```python
from build123d import *

# Parameters (mm, degrees)
SKETCH_1_W          = 123
SKETCH_1_H          = 80
EXTRUDE_1_DEPTH     = 93
SHELL_1_T           = -3
SKETCH_2_W          = 50
SKETCH_2_H          = 117
CUT_EXTRUDE_1_DEPTH = 138.227001716
FILLET_1_R          = 5
FILLET_2_R          = 5
CUT_EXTRUDE_2_REACH = 161.305
CUT_EXTRUDE_4_REACH = 161.305
SKETCH_5_W          = 30
SKETCH_5_H          = 56
CUT_EXTRUDE_5_REACH = 120.454
SKETCH_6_R          = 10
FILLET_3_R          = 5
CUT_EXTRUDE_6_REACH = 120.454
SKETCH_7_W          = 5
SKETCH_7_H          = 28


with BuildPart() as part:
    # 草圖1 → 填料-伸長1 (new body)
    with BuildSketch(Plane(origin=(0, 0, 0), x_dir=(0, 0, -1), z_dir=(1, 0, 0))):
        Rectangle(SKETCH_1_W, SKETCH_1_H)
    extrude(amount=EXTRUDE_1_DEPTH)

    # 薄殼1
    shell_1_openings = [part.faces().sort_by_distance(p)[0] for p in [
        (93, 0, 0),
    ]]
    offset(amount=SHELL_1_T, openings=shell_1_openings, kind=Kind.INTERSECTION)

    # 草圖2 → 除料-伸長1 (cut, through all)
    with BuildSketch(Plane(origin=(0, 40, 0), x_dir=(1, 0, 0), z_dir=(0, 1, 0))):
        with Locations((68, 0)):
            Rectangle(SKETCH_2_W, SKETCH_2_H)
    extrude(amount=-CUT_EXTRUDE_1_DEPTH, mode=Mode.SUBTRACT)

    # 圓角1
    fillet_1_edges = [part.edges().sort_by_distance(p)[0] for p in [
        (0, -40, 0),
        (0, 40, 0),
    ]]
    fillet(fillet_1_edges, radius=FILLET_1_R)

    # 圓角2
    fillet_2_edges = [part.edges().sort_by_distance(p)[0] for p in [
        (93, -40, 60),
        (93, -40, -60),
        (93, 40, 60),
        (93, 40, -60),
    ]]
    fillet(fillet_2_edges, radius=FILLET_2_R)

    # 草圖3 → 除料-伸長2 (cut, up to next)
    with BuildSketch(Plane(origin=(0, 0, -61.5), x_dir=(-1, 0, 0), z_dir=(0, 0, -1)), mode=Mode.PRIVATE) as cut_extrude_2_sk1:
        with BuildLine():
            Line((-76.5, -25), (-76.5, 25))
            ThreePointArc((-76.5, 25), (-74, 27.5), (-71.5, 25))
            Line((-71.5, 25), (-71.5, -25))
            ThreePointArc((-71.5, -25), (-74, -27.5), (-76.5, -25))
        make_face()
    cut_extrude_2_tool1 = extrude(cut_extrude_2_sk1.sketch, amount=-CUT_EXTRUDE_2_REACH, mode=Mode.PRIVATE) & part.part
    cut_extrude_2 = cut_extrude_2_tool1.solids().sort_by_distance((74, 0, -61.5))[0]
    add(cut_extrude_2, mode=Mode.SUBTRACT)

    # 鏡射1: 除料-伸長2 across plane
    add(cut_extrude_2.mirror(Plane.XY), mode=Mode.SUBTRACT)

    # 草圖5 → 除料-伸長4 (cut, up to next)
    with BuildSketch(Plane(origin=(0, 0, -61.5), x_dir=(-1, 0, 0), z_dir=(0, 0, -1)), mode=Mode.PRIVATE) as cut_extrude_4_sk1:
        with Locations((-38, 2)):
            Rectangle(SKETCH_5_W, SKETCH_5_H)
    cut_extrude_4_tool1 = extrude(cut_extrude_4_sk1.sketch, amount=-CUT_EXTRUDE_4_REACH, mode=Mode.PRIVATE) & part.part
    add(cut_extrude_4_tool1.solids().sort_by_distance((38, 2, -61.5))[0], mode=Mode.SUBTRACT)

    # 草圖6 → 除料-伸長5 (cut, up to next)
    with BuildSketch(Plane.ZY, mode=Mode.PRIVATE) as cut_extrude_5_sk1:
        with Locations((41.5, 20)):
            Circle(SKETCH_6_R)
    cut_extrude_5_tool1 = extrude(cut_extrude_5_sk1.sketch, amount=-CUT_EXTRUDE_5_REACH, mode=Mode.PRIVATE) & part.part
    add(cut_extrude_5_tool1.solids().sort_by_distance((0, 20, 41.5))[0], mode=Mode.SUBTRACT)

    # 圓角3
    fillet_3_edges = [part.edges().sort_by_distance(p)[0] for p in [
        (23, -26, -60),
        (23, 30, -60),
        (53, 30, -60),
        (53, -26, -60),
    ]]
    fillet(fillet_3_edges, radius=FILLET_3_R)

    # 草圖7 → 除料-伸長6 (cut, up to next)
    with BuildSketch(Plane.ZY, mode=Mode.PRIVATE) as cut_extrude_6_sk1:
        with Locations((1, 18)):
            Rectangle(SKETCH_7_W, SKETCH_7_H)
    cut_extrude_6_tool1 = extrude(cut_extrude_6_sk1.sketch, amount=-CUT_EXTRUDE_6_REACH, mode=Mode.PRIVATE) & part.part
    add(cut_extrude_6_tool1.solids().sort_by_distance((0, 18, 1))[0], mode=Mode.SUBTRACT)


solid = part.part
```
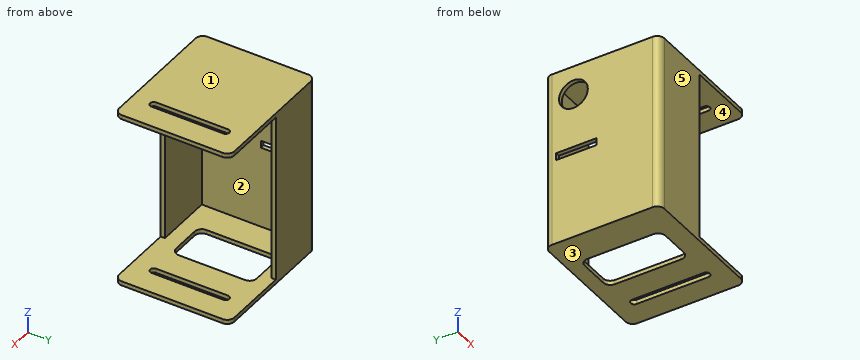
Read the model definition and answer for the solid it produces. Units are mm, in the model's axes. Face numbers are marked on the shaded views. A direction names the side the tool comes from. Give positions to 0.01 mm unless a question says otherwise; leave off trailing zeros. Order: outer loops, then holes, each group sorted by start corner. A loop starts at its lowest first (then second) coordinate and runs counter-clockwise, first axis right, second up.
(1) Find section D-D (y = 20). Give the vertices of the cut face in (x, z), plus the area to 3 significant figures.
(2) Find section C-C (x = 57.5). Give the vertices of the cut face in (y, z).
(3) Straight lines are drawn through the part: L1, parallel to Y at x = 26, z = 53; L2, parallel to Z at x = 23, y = -26.5; L3, parallel to X at y = 0, z = -40.5. For each, find the intervals that lie inside material, in ascending order.
(4) Find section A-A (z = 41.5). Give the vertices of the cut face in (x, y).
(5) Find section B-B (y = 5.5). Give the vertices of the cut face in (x, z).
(6) For the marked faces 1 and 2, determine the directions among +Z, -Z, +X, -X, +Y, -Y from which every point of the face is accessible in a straight line to the end or side of a thin tool.
(7) Given pin 1 (22 mm diameter, centred on y = -17, z = -22.5, fed in from +X); pin 2 (0.9 mm diameter, centred on y = -38, z = 19, fed in from +X); pin 3 (3.5 mm diameter, centred on x = 1.5, z = 0.5, fed in from -Y), each flat-ended and moving along its own axis, determine where each tip first touches the part or whether it passes through.
(8) For a pull along Z with two mould halves and no side action, classify the marked faces 3, 4 and 5 as released by +Z, released by -Z, zero draft, split by the parting line, or undercut.
Result sheet:
1. outline: (0, -61.5) - (23, -61.5) - (23, -58.5) - (3, -58.5) - (3, -1.5) - (0, -1.5) - close; (0, 3.5) - (3, 3.5) - (3, 31.5) - (0, 31.5) - close; (0, 51.5) - (3, 51.5) - (3, 58.5) - (71.5, 58.5) - (71.5, 61.5) - (0, 61.5) - close; (53, -61.5) - (71.5, -61.5) - (71.5, -58.5) - (53, -58.5) - close; (76.5, -61.5) - (93, -61.5) - (93, -58.5) - (76.5, -58.5) - close; (76.5, 58.5) - (93, 58.5) - (93, 61.5) - (76.5, 61.5) - close
1. area: 714 mm2
2. outline: (-40, -61.5) - (40, -61.5) - (40, -58.5) - (-40, -58.5) - close; (-40, 58.5) - (40, 58.5) - (40, 61.5) - (-40, 61.5) - close
3. L1: y = -40 to -37, 37 to 40
3. L2: z = -61.5 to -58.5, 58.5 to 61.5
3. L3: x = 0 to 3
4. outline: (0, -35) arc R5 ccw to (5, -40) - (43, -40) - (43, -37) - (3, -37) - (3, 10) - (0, 10) - close; (0, 30) - (3, 30) - (3, 37) - (43, 37) - (43, 40) - (5, 40) arc R5 ccw to (0, 35) - close
5. outline: (0, -61.5) - (23, -61.5) - (23, -58.5) - (3, -58.5) - (3, -1.5) - (0, -1.5) - close; (0, 3.5) - (3, 3.5) - (3, 58.5) - (71.5, 58.5) - (71.5, 61.5) - (0, 61.5) - close; (53, -61.5) - (71.5, -61.5) - (71.5, -58.5) - (53, -58.5) - close; (76.5, -61.5) - (93, -61.5) - (93, -58.5) - (76.5, -58.5) - close; (76.5, 58.5) - (93, 58.5) - (93, 61.5) - (76.5, 61.5) - close
6. face 1: +Z, +X, -X, +Y, -Y
6. face 2: +X
7. pin 1: stops at x = 3
7. pin 2: stops at x = 43
7. pin 3: stops at y = -39.68
8. face 3: released by -Z
8. face 4: undercut
8. face 5: zero draft
